from build123d import *

# Parameters (mm, degrees)
F0_W     = 20
F0_H     = 20
F1_DEPTH = 15
F3_DEPTH = 10


with BuildPart() as f1:
    # F0 (on Right) → F1 (new body, symmetric)
    with BuildSketch(Plane.YZ):
        with Locations((-10, 10)):
            Rectangle(F0_W, F0_H)
    extrude(amount=F1_DEPTH, both=True)

    # F2 (on Right) → F3 (cut, symmetric)
    with BuildSketch(Plane.YZ):
        Polygon((-20, 5), (0, 20), (-20, 20), align=None)
    extrude(amount=F3_DEPTH, both=True, mode=Mode.SUBTRACT)


solid = f1.part
Input: part model. Units: mm. Frame: model coordinates. A direction names the side the tool comes from. Give positions to 0.01 mm unless a question says otherwise; leave off trailing zeros. Order: outer loops, then holes, each group sorted by start corner. A loop starts at its lowest first (then second) coordinate and runs counter-clockwise, first axis right, second up. Notation, with made-up numbers: M 61,2 L 65,2 A33 cw 65,32 Z; hole C -6.5,86.25 d11. An arc over 180 degrees is marked long. Answer as a JSON object with one key per item and string values.
1. Cut plane B-B, the plane z = 11.75. Output: boundary loops of the cut face in (x, y).
Result sheet:
{"outline": "M -15,-20 L -10,-20 L -10,-11 L 10,-11 L 10,-20 L 15,-20 L 15,0 L -15,0 Z"}
2. Pull-direction query (X, two-part tool) for faces 1 (the flat face through (-10, -12, 14)), 2 (the flat face through (15, -10, 10)), 3 (the flat face through (4, -20, 3)); classes: +X half, -X half, draft (parallel to the pull), parting line (faces both ways), or undercut.
Result sheet:
{"face 1": "undercut", "face 2": "+X half", "face 3": "draft"}
3. Cut plane C-C, the plane x = -9. Output: boundary loops of the cut face in (y, z), and give its area (3 significant figures).
Result sheet:
{"outline": "M -20,0 L 0,0 L 0,20 L -20,5 Z", "area": "250 mm²"}
4. First-contact query: P1, Ø3, axis at x = 3, z = 14.5, coming from the -Y side. Flat tip, straight axial feed; report the tip coordinate or a pass-through.
Result sheet:
{"P1": "y = -9.33"}
5. Reachability of faces 4 (the flat face through (0.14, -10.14, 12.395)), 5 (the flat face through (0, -10, 0)) from +Z, -Z, +X, -X, +Y, -Y: full face, straight path, thin tool, end or side. Return the list, or none.
Result sheet:
{"face 4": "+Z, -Y", "face 5": "-Z, +X, -X, +Y, -Y"}
6. Ray query, line 1 (X direction, y = -10, z = 14); line 2 (Y direction, x = 0, z = 12.5); line 3 (Y direction, x = -5.75, z = 5.75). Return the intervals inside material, ascending. Write a range as [from, to].
Result sheet:
{"line 1": "[-15, -10], [10, 15]", "line 2": "[-10, 0]", "line 3": "[-19, 0]"}
7. Cut plane A-A, the plane y = -3. Output: boundary loops of the cut face in (x, z), and give its area (3 significant figures).
Result sheet:
{"outline": "M -15,0 L 15,0 L 15,20 L 10,20 L 10,17.75 L -10,17.75 L -10,20 L -15,20 Z", "area": "555 mm²"}
